from build123d import *

# Parameters (mm, degrees)
BOSS_EXTRUDE1_DEPTH     = 20
CUT_EXTRUDE1_REACH      = 22
SKETCH2_R               = 6.6
SKETCH2_R_2             = 1.6
SKETCH2_R_3             = 2.6
SKETCH3_R               = 11.25
CUT_EXTRUDE2_DEPTH      = 2.35
SKETCH4_R               = 7
CUT_EXTRUDE3_DEPTH      = 5.25
CUT_EXTRUDE4_DEPTH      = 6
CUT_EXTRUDE5_DEPTH      = 5.25
BOSS_EXTRUDE2_REACH     = 40.5
SKETCH10_R              = 3
BOSS_EXTRUDE3_REACH     = 41
SKETCH8_R               = 1.1
CUT_EXTRUDE6_DEPTH      = 40
SKETCH14_R              = 2.25
CUT_EXTRUDE7_DEPTH      = 5
SKETCH15_R              = 1.6
CUT_EXTRUDE8_DEPTH      = 13
CUT_EXTRUDE9_DEPTH      = 9.5
CUT_EXTRUDE9_DEPTH_BACK = 1.5
BOSS_EXTRUDE4_REACH     = 17.75
SKETCH17_W              = 1.481378883
SKETCH17_H              = 0.6
SKETCH17_W_2            = 5.287146776
SKETCH17_W_3            = 2.276797121


with BuildPart() as part:
    # Sketch1 → Boss-Extrude1 (new body)
    with BuildSketch(Plane(origin=(0, 0, 0), x_dir=(1, 0, 0), z_dir=(0, 1, 0))):
        with BuildLine():
            Line((4, -21), (17, -21))
            Line((17, -21), (17, -7.745966692))
            ThreePointArc((17, -7.745966692), (22.967354114, 0.721989217), (15.575, 7.979309181))
            ThreePointArc((15.575, 7.979309181), (-15.882243174, 7.348765322), (4, -17.036725037))
            Line((4, -17.036725037), (4, -21))
        make_face()
    extrude(amount=BOSS_EXTRUDE1_DEPTH)

    # Sketch2 → Cut-Extrude1 (cut, up to next)
    with BuildSketch(Plane(origin=(0, 20, 0), x_dir=(1, 0, 0), z_dir=(0, 1, 0)), mode=Mode.PRIVATE) as cut_extrude1_sk1:
        Circle(SKETCH2_R)
    cut_extrude1_tool1 = extrude(cut_extrude1_sk1.sketch, amount=-CUT_EXTRUDE1_REACH, mode=Mode.PRIVATE) & part.part
    add(cut_extrude1_tool1.solids().sort_by_distance((0, 20, 0))[0], mode=Mode.SUBTRACT)
    # Sketch2 → Cut-Extrude1 (cut, up to next)
    with BuildSketch(Plane(origin=(0, 20, 0), x_dir=(1, 0, 0), z_dir=(0, 1, 0)), mode=Mode.PRIVATE) as cut_extrude1_sk2:
        with Locations((-9.899494937, 9.899494937)):
            Circle(SKETCH2_R_2)
    cut_extrude1_tool2 = extrude(cut_extrude1_sk2.sketch, amount=-CUT_EXTRUDE1_REACH, mode=Mode.PRIVATE) & part.part
    add(cut_extrude1_tool2.solids().sort_by_distance((-9.899495, 20, -9.899495))[0], mode=Mode.SUBTRACT)
    # Sketch2 → Cut-Extrude1 (cut, up to next)
    with BuildSketch(Plane(origin=(0, 20, 0), x_dir=(1, 0, 0), z_dir=(0, 1, 0)), mode=Mode.PRIVATE) as cut_extrude1_sk3:
        with Locations((-9.899494937, -9.899494937)):
            Circle(SKETCH2_R_2)
    cut_extrude1_tool3 = extrude(cut_extrude1_sk3.sketch, amount=-CUT_EXTRUDE1_REACH, mode=Mode.PRIVATE) & part.part
    add(cut_extrude1_tool3.solids().sort_by_distance((-9.899495, 20, 9.899495))[0], mode=Mode.SUBTRACT)
    # Sketch2 → Cut-Extrude1 (cut, up to next)
    with BuildSketch(Plane(origin=(0, 20, 0), x_dir=(1, 0, 0), z_dir=(0, 1, 0)), mode=Mode.PRIVATE) as cut_extrude1_sk4:
        with Locations((15, 0)):
            Circle(SKETCH2_R_3)
    cut_extrude1_tool4 = extrude(cut_extrude1_sk4.sketch, amount=-CUT_EXTRUDE1_REACH, mode=Mode.PRIVATE) & part.part
    add(cut_extrude1_tool4.solids().sort_by_distance((15, 20, 0))[0], mode=Mode.SUBTRACT)
    # Sketch2 → Cut-Extrude1 (cut, up to next)
    with BuildSketch(Plane(origin=(0, 20, 0), x_dir=(1, 0, 0), z_dir=(0, 1, 0)), mode=Mode.PRIVATE) as cut_extrude1_sk5:
        with BuildLine():
            Line((8.899494937, -21), (8.899494937, 8.650495337))
            ThreePointArc((8.899494937, 8.650495337), (9.899494937, 11.499494937), (10.899494937, 8.650495337))
            Line((10.899494937, 8.650495337), (10.899494937, -21))
            Line((10.899494937, -21), (8.899494937, -21))
        make_face()
    cut_extrude1_tool5 = extrude(cut_extrude1_sk5.sketch, amount=-CUT_EXTRUDE1_REACH, mode=Mode.PRIVATE) & part.part
    add(cut_extrude1_tool5.solids().sort_by_distance((9.899495, 20, 4.346591))[0], mode=Mode.SUBTRACT)

    # Sketch3 → Cut-Extrude2 (cut)
    with BuildSketch(Plane(origin=(0, 20, 0), x_dir=(1, 0, 0), z_dir=(0, 1, 0))):
        Circle(SKETCH3_R)
    extrude(amount=-CUT_EXTRUDE2_DEPTH, mode=Mode.SUBTRACT)

    # Sketch4 → Cut-Extrude3 (cut)
    with BuildSketch(Plane(origin=(0, 17.65, 0), x_dir=(1, 0, 0), z_dir=(0, 1, 0))):
        Circle(SKETCH4_R)
    extrude(amount=-CUT_EXTRUDE3_DEPTH, mode=Mode.SUBTRACT)

    # Sketch5 → Cut-Extrude4 (cut)
    with BuildSketch(Plane(origin=(0, 20, 0), x_dir=(1, 0, 0), z_dir=(0, 1, 0))):
        Polygon((19.100505063, 2.367427702), (15, 4.734855404), (10.899494937, 2.367427702), (10.899494937, -2.367427702), (15, -4.734855404), (19.100505063, -2.367427702), align=None)
    extrude(amount=-CUT_EXTRUDE4_DEPTH, mode=Mode.SUBTRACT)

    # Sketch6 → Cut-Extrude5 (cut)
    with BuildSketch(Plane(origin=(0, 4.25, 0), x_dir=(1, 0, 0), z_dir=(0, 1, 0))):
        with BuildLine():
            Line((15, 8.5), (23.5, 8.5))
            Line((23.5, 8.5), (23.5, 0))
            Line((23.5, 0), (23.5, -8.5))
            Line((23.5, -8.5), (15, -8.5))
            ThreePointArc((15, -8.5), (10.626786079, -7.288689869), (7.5, -4))
            Line((7.5, -4), (5, -4))
            Line((5, -4), (5, 0))
            Line((5, 0), (5, 4))
            Line((5, 4), (7.5, 4))
            ThreePointArc((7.5, 4), (10.626786079, 7.288689869), (15, 8.5))
        make_face()
    extrude(amount=CUT_EXTRUDE5_DEPTH, mode=Mode.SUBTRACT)

    # Sketch10 → Boss-Extrude2 (add, up to next)
    with BuildSketch(Plane.XY.offset(21), mode=Mode.PRIVATE) as boss_extrude2_sk1:
        with Locations((5.75, 6.5)):
            Circle(SKETCH10_R)
    boss_extrude2_tool1 = extrude(boss_extrude2_sk1.sketch, amount=-BOSS_EXTRUDE2_REACH, mode=Mode.PRIVATE) - part.part
    add(boss_extrude2_tool1.solids().sort_by_distance((5.75, 6.5, 21))[0])

    # Sketch11 → Boss-Extrude3 (add, up to next)
    with BuildSketch(Plane.XY.offset(-18), mode=Mode.PRIVATE) as boss_extrude3_sk1:
        Polygon((-1.005553499, 6.5), (2.74722325, 0), (10.25277675, 0), (14.005553499, 6.5), (10.25277675, 13), (2.74722325, 13), align=None)
    boss_extrude3_tool1 = extrude(boss_extrude3_sk1.sketch, amount=BOSS_EXTRUDE3_REACH, mode=Mode.PRIVATE) - part.part
    add(boss_extrude3_tool1.solids().sort_by_distance((6.5, 6.5, -18))[0])

    # Sketch8 → Cut-Extrude6 (cut, through all)
    with BuildSketch(Plane.XY.offset(21)):
        with Locations((6.399494937, 6.5)):
            Circle(SKETCH8_R)
    extrude(amount=-CUT_EXTRUDE6_DEPTH, mode=Mode.SUBTRACT)

    # Sketch13 → Cut-Revolve1 (revolve, cut)
    with BuildSketch(Plane.ZY.offset(-6.5)):
        Polygon((-6, 6.5), (-4, 6.5), (-4, 8.678199262), (-6, 7), align=None)
    revolve(axis=Axis((6.5, 6.5, -18), (0, 0, 1)), mode=Mode.SUBTRACT)

    # Sketch14 → Cut-Extrude7 (cut)
    with BuildSketch(Plane(origin=(0, 0, -18), x_dir=(-1, 0, 0), z_dir=(0, 0, -1))):
        with Locations((-6.399494937, 6.5)):
            Circle(SKETCH14_R)
    extrude(amount=-CUT_EXTRUDE7_DEPTH, mode=Mode.SUBTRACT)

    # Sketch15 → Cut-Extrude8 (cut)
    with BuildSketch(Plane(origin=(17, 0, 0), x_dir=(0, 0, -1), z_dir=(1, 0, 0))):
        with Locations((-17, 12)):
            Circle(SKETCH15_R)
    extrude(amount=-CUT_EXTRUDE8_DEPTH, mode=Mode.SUBTRACT)

    # Sketch16 → Cut-Extrude9 (cut, two sides)
    with BuildSketch(Plane.ZY.offset(-4)) as cut_extrude9_sk:
        Polygon((20.233161507, 12), (18.616580754, 14.8), (15.383419246, 14.8), (13.766838493, 12), (15.383419246, 9.2), (18.616580754, 9.2), align=None)
    extrude(amount=CUT_EXTRUDE9_DEPTH, mode=Mode.SUBTRACT)
    extrude(cut_extrude9_sk.sketch, amount=-CUT_EXTRUDE9_DEPTH_BACK, mode=Mode.SUBTRACT)

    # Sketch17 → Boss-Extrude4 (add, up to next)
    with BuildSketch(Plane(origin=(0, 4.25, 0), x_dir=(1, 0, 0), z_dir=(0, 1, 0)), mode=Mode.PRIVATE) as boss_extrude4_sk1:
        with Locations((11.640184379, 0.05)):
            Rectangle(SKETCH17_W, SKETCH17_H)
    boss_extrude4_tool1 = extrude(boss_extrude4_sk1.sketch, amount=BOSS_EXTRUDE4_REACH, mode=Mode.PRIVATE) - part.part
    add(boss_extrude4_tool1.solids().sort_by_distance((11.640184, 4.25, -0.05))[0])
    # Sketch17 → Boss-Extrude4 (add, up to next)
    with BuildSketch(Plane(origin=(0, 4.25, 0), x_dir=(1, 0, 0), z_dir=(0, 1, 0)), mode=Mode.PRIVATE) as boss_extrude4_sk2:
        Polygon((22.23765915, 3.330781542), (10.899494937, 3.330781542), (10.899494937, 2.730781542), (22.440052992, 2.730781542), align=None)
    boss_extrude4_tool2 = extrude(boss_extrude4_sk2.sketch, amount=BOSS_EXTRUDE4_REACH, mode=Mode.PRIVATE) - part.part
    add(boss_extrude4_tool2.solids().sort_by_distance((16.619325, 4.25, -3.029897))[0])
    # Sketch17 → Boss-Extrude4 (add, up to next)
    with BuildSketch(Plane(origin=(0, 4.25, 0), x_dir=(1, 0, 0), z_dir=(0, 1, 0)), mode=Mode.PRIVATE) as boss_extrude4_sk3:
        Polygon((22.477954877, -2.64697567), (10.899494937, -2.64697567), (10.899494937, -3.24697567), (22.217055012, -3.24697567), align=None)
    boss_extrude4_tool3 = extrude(boss_extrude4_sk3.sketch, amount=BOSS_EXTRUDE4_REACH, mode=Mode.PRIVATE) - part.part
    add(boss_extrude4_tool3.solids().sort_by_distance((16.623748, 4.25, 2.945836))[0])
    # Sketch17 → Boss-Extrude4 (add, up to next)
    with BuildSketch(Plane(origin=(0, 4.25, 0), x_dir=(1, 0, 0), z_dir=(0, 1, 0)), mode=Mode.PRIVATE) as boss_extrude4_sk4:
        Polygon((20.100469452, -6), (10.899494937, -6), (10.899494937, -6.6), (19.187050839, -6.6), align=None)
    boss_extrude4_tool4 = extrude(boss_extrude4_sk4.sketch, amount=BOSS_EXTRUDE4_REACH, mode=Mode.PRIVATE) - part.part
    add(boss_extrude4_tool4.solids().sort_by_distance((15.275603, 4.25, 6.294777))[0])
    # Sketch17 → Boss-Extrude4 (add, up to next)
    with BuildSketch(Plane(origin=(0, 4.25, 0), x_dir=(1, 0, 0), z_dir=(0, 1, 0)), mode=Mode.PRIVATE) as boss_extrude4_sk5:
        with Locations((20.290372632, 0.05)):
            Rectangle(SKETCH17_W_2, SKETCH17_H)
    boss_extrude4_tool5 = extrude(boss_extrude4_sk5.sketch, amount=BOSS_EXTRUDE4_REACH, mode=Mode.PRIVATE) - part.part
    add(boss_extrude4_tool5.solids().sort_by_distance((20.290373, 4.25, -0.05))[0])
    # Sketch17 → Boss-Extrude4 (add, up to next)
    with BuildSketch(Plane(origin=(0, 4.25, 0), x_dir=(1, 0, 0), z_dir=(0, 1, 0)), mode=Mode.PRIVATE) as boss_extrude4_sk6:
        Polygon((10.899494937, 6.25), (10.899494937, 5.65), (20.530479048, 5.65), (19.895586914, 6.25), align=None)
    boss_extrude4_tool6 = extrude(boss_extrude4_sk6.sketch, amount=BOSS_EXTRUDE4_REACH, mode=Mode.PRIVATE) - part.part
    add(boss_extrude4_tool6.solids().sort_by_distance((15.558067, 4.25, -5.946592))[0])
    # Sketch17 → Boss-Extrude4 (add, up to next)
    with BuildSketch(Plane(origin=(0, 4.25, 0), x_dir=(1, 0, 0), z_dir=(0, 1, 0)), mode=Mode.PRIVATE) as boss_extrude4_sk7:
        Polygon((8.899494937, -3.24697567), (8.899494937, -2.64697567), (6.922653913, -2.64697567), (6.045950695, -2.64697567), (5.800562103, -3.24697567), (7.144610194, -3.24697567), align=None)
    boss_extrude4_tool7 = extrude(boss_extrude4_sk7.sketch, amount=BOSS_EXTRUDE4_REACH, mode=Mode.PRIVATE) - part.part
    add(boss_extrude4_tool7.solids().sort_by_distance((7.410533, 4.25, 2.951098))[0])
    # Sketch17 → Boss-Extrude4 (add, up to next)
    with BuildSketch(Plane(origin=(0, 4.25, 0), x_dir=(1, 0, 0), z_dir=(0, 1, 0)), mode=Mode.PRIVATE) as boss_extrude4_sk8:
        Polygon((8.899494937, 3.330781542), (7.179776581, 3.330781542), (5.759276556, 3.330781542), (6.078412351, 2.730781542), (6.950600509, 2.730781542), (8.899494937, 2.730781542), align=None)
    boss_extrude4_tool8 = extrude(boss_extrude4_sk8.sketch, amount=BOSS_EXTRUDE4_REACH, mode=Mode.PRIVATE) - part.part
    add(boss_extrude4_tool8.solids().sort_by_distance((7.407746, 4.25, -3.036135))[0])
    # Sketch17 → Boss-Extrude4 (add, up to next)
    with BuildSketch(Plane(origin=(0, 4.25, 0), x_dir=(1, 0, 0), z_dir=(0, 1, 0)), mode=Mode.PRIVATE) as boss_extrude4_sk9:
        with Locations((7.761096377, 0.05)):
            Rectangle(SKETCH17_W_3, SKETCH17_H)
    boss_extrude4_tool9 = extrude(boss_extrude4_sk9.sketch, amount=BOSS_EXTRUDE4_REACH, mode=Mode.PRIVATE) - part.part
    add(boss_extrude4_tool9.solids().sort_by_distance((7.761096, 4.25, -0.05))[0])


solid = part.part
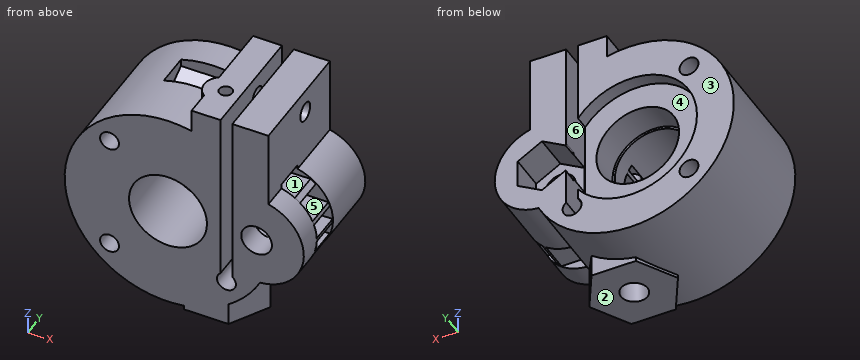
The listing builds one solid part. Answer for the finished solid, in the listing's coordinates (mm). Face numbers are marked on the shaded views. A direction names the side the tool comes from. Round coordinates to 2 decimals unless told otherwise and drop trailing zeros. Write each loop counter-clockwise with the first axis right and the second up, starting at its lowest first coordinate (ties: lowest second). Pieces come first, ordered by that corner, then holes. Notation, with made-up numbers: (-32, 44.25) - (22, 44.25) arc R23 cw to (22, 75.25) - close; hole circle Ø10 at (45, 12). An arc over 180 degrees is marked (long way). Use one line per item in the form item = value. Start each with the question number.
Item 1: A cutting plane is placed at B-B (x = -3). Write down the section's boundary in (y, z).
Item 2: A tool of negligible diameter and unlimited length cuts with its end or side. For the marked faces 4, 5 and 6, from which of +Z, -Z, +X, -X, +Y, -Y can it reach the whole face along a straight path? Write none if from no direction.
Item 3: Flat-ended cylindrical pins translate along their axes: pin 1 Ø1.6 at (x, y) = (21, 7) entering from -Z; pin 2 Ø1.1 at (x, y) = (8, 6.5) entering from -Z; pin 3 Ø8 at (y, z) = (8.5, -6) entering from +X; pin 4 Ø6 at (x, z) = (12.5, -3) entering from -Y. Find the tip coordinate at first contact, or state that the pin passes through.
Item 4: A cutting plane is placed at A-A (z = 13). Write down the section's boundary in (x, y), plus the area to 3 significant figures.
Item 5: A cutting plane is placed at C-C (y = 6). Give the number of separate pieces and of enclosed holes in the cut face, plus the area to 3 significant figures.
Item 6: Determine the mould class of the marked faces 1, 2 and 3 for opening direction Z: +Z half, -Z half, draft (parallel to the pull), parting line (faces both ways), or undercut.
Item 7: Find the intervals of material crossed by line 1 (X direction, y = 14.6, z = 0); line 2 (X direction, y = 10.25, z = 0); line 3 (X direction, y = 4.5, z = 0), in increasing order. Write a range as [from, to].
The answers:
q1.outline = (0, -17.24) - (20, -17.24) - (20, -10.84) - (17.65, -10.84) - (17.65, -6.32) - (12.4, -6.32) - (12.4, -5.88) - (0, -5.88) - close; (0, 5.88) - (12.4, 5.88) - (12.4, 6.32) - (17.65, 6.32) - (17.65, 10.84) - (20, 10.84) - (20, 17.24) - (14.8, 17.24) - (14.8, 15.38) - (12, 13.77) - (9.2, 15.38) - (9.2, 17.24) - (0, 17.24) - close
q2.face_4 = +Y
q2.face_5 = +X
q2.face_6 = +Z, +Y, -Y
q3.pin_1 = -5.96
q3.pin_2 = -13
q3.pin_3 = 22.71
q3.pin_4 = 0
q4.outline = (-11.72, 0) - (8.9, 0) - (8.9, 20) - (-11.72, 20) - close; (10.9, 0) - (17, 0) - (17, 20) - (10.9, 20) - close; hole circle Ø2.2 at (6.4, 6.5)
q4.area = 531 mm^2
q5.separate_pieces = 13
q5.enclosed_holes = 2
q5.area = 720 mm^2
q6.face_1 = undercut
q6.face_2 = -Z half
q6.face_3 = draft
q7.line_1 = [-17.5, -7], [7, 8.9], [19.1, 23]
q7.line_2 = [-17.5, -6.6], [6.6, 8.9], [10.9, 12.4], [17.6, 23]
q7.line_3 = [-17.5, -6.6], [6.62, 8.9], [10.9, 12.38], [17.65, 22.93]
